```python
from build123d import *

# Parameters (mm, degrees)
SKETCH_1_R          = 3
SKETCH_1_R_2        = 4.6
EXTRUDE_1_DEPTH     = 6
SKETCH_3_R          = 7
CUT_EXTRUDE_1_DEPTH = 3
FILLET_1_R          = 20


with BuildPart() as part:
    # ｽｹｯﾁ1 → ﾎﾞｽ - 押し出し1 (new body)
    with BuildSketch(Plane(origin=(0, 0, 0), x_dir=(1, 0, 0), z_dir=(0, 1, 0))):
        with BuildLine():
            Line((-17.25, 6), (17.25, 6))
            ThreePointArc((17.25, 6), (23.25, 0), (17.25, -6))
            Line((17.25, -6), (-17.25, -6))
            ThreePointArc((-17.25, -6), (-23.25, 0), (-17.25, 6))
        make_face()
        with Locations((-17.25, 0)):
            Circle(SKETCH_1_R, mode=Mode.SUBTRACT)
        with Locations((17.25, 0)):
            Circle(SKETCH_1_R_2, mode=Mode.SUBTRACT)
    extrude(amount=EXTRUDE_1_DEPTH)

    # ｽｹｯﾁ3 → ｶｯﾄ - 押し出し1 (cut)
    with BuildSketch(Plane(origin=(0, 6, 0), x_dir=(1, 0, 0), z_dir=(0, 1, 0))):
        with Locations((17.25, 0)):
            Circle(SKETCH_3_R)
    extrude(amount=-CUT_EXTRUDE_1_DEPTH, mode=Mode.SUBTRACT)

    # ﾌｨﾚｯﾄ1
    fillet_1_edges = [part.edges().sort_by_distance(p)[0] for p in [
        (13.644448725, 4.5, -6),
    ]]
    fillet(fillet_1_edges, radius=FILLET_1_R)


solid = part.part
```
Model file for the job. Use its own axes, mm. A direction names the side the tool comes from. Coordinates: 2 decimals unless noted, no trailing zeros. Loops run counter-clockwise (first coordinate to the right, second up) from the corner with the lowest first, then second, coordinate; pieces in that order, holes last. Notation, with made-up numbers: (83.25, 88) - (142.25, 88) arc R8 ccw to (142.25, 96) - close; hole circle Ø2 at (73.25, 11). An arc over 180 degrees is marked (long way). Write item = value, one per line. Start each with the question number.
Item 1: Pull direction X, two halves, no side cores. Call faces 1 (the face through (0, 3, 6)), 2 (the face through (3.851, 4.521, -3.497)), 3 (the face through (12.654, 1.479, -0.202)): +X half, -X half, draft (parallel to the pull), parting line (faces both ways), or undercut.
Item 2: Drop flat-ended pins along their axis: pin 1 Ø5 at (x, z) = (16, 3) entering from -Y; pin 2 Ø1 at (x, z) = (16, 2.5) entering from -Y; pin 3 Ø3 at (y, z) = (2.5, 4) entering from +X. Give the stop position or say it passes through.
Item 3: Saw through at D-D, the plane x = 2. List the corners of the cut face in (y, z), then the cut area to 3 significant figures.
Item 4: Saw through at C-C, the plane y = 2.4. List the corners of the cut face in (x, z), then the cut area to 3 significant figures.
Item 5: Saw through at B-B, the plane z = 0. List the corners of the cut face in (x, y), then the cut area to 3 significant figures.
Item 6: 3-axis set-ups, long thin cutter, end or side, ignore diameter. For faces 4 (the face through (12, 3, -1)), 5 (the face through (-4, 2, -6)): which of +Z, -Z, +X, -X, +Y, -Y reach the whole face in a straight line?
Item 7: Saw through at A-A, the plane x = 15. List the corners of the cut face in (y, z), then the cut area to 3 significant figures.
Item 8: Wall check: probe 1 along X at (y, z) = (2.25, -0.25); probe 2 along Z at (x, y) = (17.25, 1.1); probe 3 along Z at (x, y) = (-17.25, 2.8). Give the ranges that are in metal, low to high. Write a range as [from, to].
Answers:
q1.face_1 = draft
q1.face_2 = +X half
q1.face_3 = undercut
q2.pin_1 = 0
q2.pin_2 = through
q2.pin_3 = 22.7
q3.outline = (0, -6) - (3, -6) - (3, -4.4) - (6, -4.4) - (6, 6) - (0, 6) - close
q3.area = 67.2 mm2
q4.outline = (-17.25, -6) - (17.25, -6) arc R6 ccw to (17.25, 6) - (-17.25, 6) arc R6 ccw to start; hole circle Ø6 at (-17.25, 0); hole circle Ø9.2 at (17.25, 0)
q4.area = 432 mm2
q5.outline = (-23.25, 0) - (-20.25, 0) - (-20.25, 6) - (-23.25, 6) - close; (-14.25, 0) - (12.65, 0) - (12.65, 3) - (8.45, 3) - (8.45, 6) - (-14.25, 6) - close; (21.85, 0) - (23.25, 0) - (23.25, 3) - (21.85, 3) - close
q5.area = 171 mm2
q6.face_4 = -Z, +X, +Y
q6.face_5 = -Z, +X, -X, +Y, -Y
q7.outline = (0, -6) - (3, -6) - (3, -4.01) - (0, -4.01) - close; (0, 4.01) - (3, 4.01) - (3, 6) - (0, 6) - close
q7.area = 11.9 mm2
q8.probe_1 = [-23.24, -20.24], [-14.26, 12.66], [21.84, 23.24]
q8.probe_2 = [-6, -4.6], [4.6, 6]
q8.probe_3 = [-6, -3], [3, 6]
